Check sheet for the modelled part. Datum: model origin and axes. Units: mm. Face numbers are marked on the shaded views. Coordinates: 2 decimals unless noted, no trailing zeros. Loops run counter-clockwise (first coordinate to the right, second up) from the corner with the lowest first, then second, coordinate; pieces in that order, holes last. Notation, with made-up numbers: M 36.5,16.5 L 86.5,16.5 A9 cw 86.5,24.5 Z; hole C 9.5,76 d8. An arc over 180 degrees is marked long. Return JSON: item names as keys, results as strings.
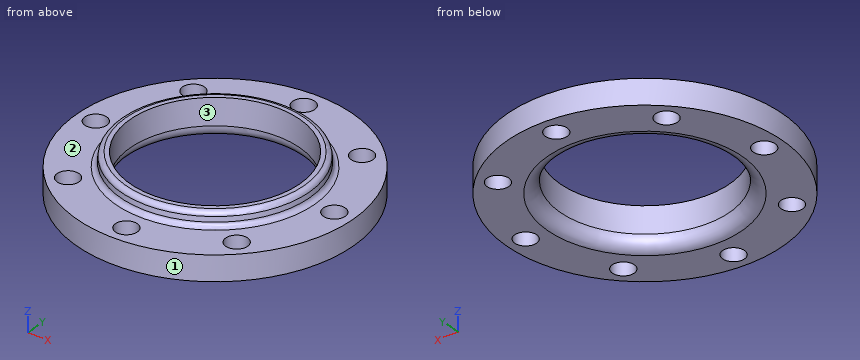
from build123d import *

# Parameters (mm, degrees)
F2_R     = 11.1
F3_DEPTH = 25.401


# Not quite as in the source:
# - a feature names something its author has since deleted; it is built from what else it names


with BuildPart() as f1:
    # F0 (on Front) → F1 (revolve)
    with BuildSketch(Plane.XZ):
        with BuildLine():
            ThreePointArc((85.75, 12.7), (89.4697438789, 3.7197438789), (98.45, 0))
            Line((98.45, 0), (139.7, 0))
            Line((139.7, 0), (139.7, 25.4))
            Line((139.7, 25.4), (100.5816558701, 25.4))
            ThreePointArc((100.5816558701, 25.4), (97.203704832, 26.7136133159), (95.6006823796, 29.9642212863))
            Line((95.6006823796, 29.9642212863), (95.1569785983, 35.0357787137))
            ThreePointArc((95.1569785983, 35.0357787137), (93.5539561459, 38.2863866841), (90.1760051078, 39.6))
            Line((90.1760051078, 39.6), (85.75, 39.6))
            Line((85.75, 39.6), (85.75, 12.7))
        make_face()
    revolve(axis=Axis((0, 0, 19.8), (0, 0, 1)))

    # F2 (on face) → F3 (cut, through all)
    with BuildSketch(Plane.XY.offset(25.4)):
        with Locations((0, 120.65)):
            Circle(F2_R)
        with Locations((-85.3124331502, 85.3124331502)):
            Circle(F2_R)
        with Locations((-120.65, 0)):
            Circle(F2_R)
        with Locations((-85.3124331502, -85.3124331502)):
            Circle(F2_R)
        with Locations((0, -120.65)):
            Circle(F2_R)
        with Locations((85.3124331502, -85.3124331502)):
            Circle(F2_R)
        with Locations((120.65, 0)):
            Circle(F2_R)
        with Locations((85.3124331502, 85.3124331502)):
            Circle(F2_R)
    extrude(amount=-F3_DEPTH, mode=Mode.SUBTRACT)


solid = f1.part
1) Go/stop test with flat-tipped pins: pin 1 Ø2 at (y, z) = (81, 12.5) entering from +X; pin 2 Ø3 at (x, z) = (-69.5, 32) entering from -Y; pin 3 Ø10 at (x, z) = (61, 23) entering from -Y; pin 4 Ø20 at (x, y) = (85.31, -85.31) entering from -Z. Record where each tip stops, or that it passes through.
Answers:
{"pin 1": "x = 114.53", "pin 2": "y = -66.96", "pin 3": "y = -127.98", "pin 4": "through"}
2) Draft check along Y on the marked faces 1, 2 and 3. Enter one of: +Y half, -Y half, draft (parallel to the pull), parting line (faces both ways), or undercut.
Answers:
{"face 1": "parting line", "face 2": "draft", "face 3": "undercut"}
3) Section check C-C on y = -120.65. Record the cut outline in (x, z).
Answers:
{"outline": "M -70.42,0 L -11.1,0 L -11.1,25.4 L -70.42,25.4 Z; M 11.1,0 L 70.42,0 L 70.42,25.4 L 11.1,25.4 Z"}
4) Section check A-A on y = 0. Record the cut outline in (x, z), then the cut area to 3 significant figures.
Answers:
{"outline": "M -139.7,0 L -131.75,0 L -131.75,25.4 L -139.7,25.4 Z; M -109.55,0 L -98.45,0 A12.7 ccw -85.75,12.7 L -85.75,39.6 L -90.18,39.6 A5 ccw -95.16,35.04 L -95.6,29.96 A5 cw -100.58,25.4 L -109.55,25.4 Z; M 85.75,12.7 A12.7 ccw 98.45,0 L 109.55,0 L 109.55,25.4 L 100.58,25.4 A5 cw 95.6,29.96 L 95.16,35.04 A5 ccw 90.18,39.6 L 85.75,39.6 Z; M 131.75,0 L 139.7,0 L 139.7,25.4 L 131.75,25.4 Z", "area": "1,820 mm²"}
5) Section check D-D on z = 3.5. Count the separate pieces of the cut face and the enclosed holes in it, then the cut area to 3 significant figures.
Answers:
{"separate pieces": "1", "enclosed holes": "9", "area": "32,900 mm²"}
6) Scan lines: line 1 along Y through (x, z) = (0, 14); line 2 along X through (y, z) = (80.5, 5); line 3 along Z through (x, y) = (-103.5, 92). Record each from-to range of solid material in increasing order. Write a range as [from, to].
Answers:
{"line 1": "[-139.7, -131.75], [-109.55, -85.75], [85.75, 109.55], [131.75, 139.7]", "line 2": "[-114.17, -95.31], [-75.31, -36.41], [36.41, 75.31], [95.31, 114.17]", "line 3": "[0, 25.4]"}
